The listing builds one solid part. Answer for the finished solid, in the listing's coordinates (mm). A direction names the side the tool comes from. Coordinates: 2 decimals unless noted, no trailing zeros. Loops run counter-clockwise (first coordinate to the right, second up) from the corner with the lowest first, then second, coordinate; pieces in that order, holes last. Notation, with made-up numbers: M 64.5,-28 L 68.5,-28 A10 ccw 68.5,-22 Z; hole C -14.5,54.5 d1. An arc over 180 degrees is marked long. Answer as CSV lines item,"result". Start each with the question number.
```python
from build123d import *

# Parameters (mm, degrees)
SKETCH2_R               = 20
BOSS_EXTRUDE1_DEPTH     = 20
SKETCH3_R               = 63.245553203
SKETCH3_R_2             = 55
CUT_EXTRUDE1_DEPTH      = 101
CUT_EXTRUDE1_DEPTH_BACK = 10


with BuildPart() as part:
    # Sketch1 → Revolve1 (revolve)
    with BuildSketch(Plane(origin=(0, 0, 0), x_dir=(1, 0, 0), z_dir=(0, 1, 0))):
        Polygon((70, -780), (70, -730), (60, -730), (60, -40), (0, -40), (0, -60), (45, -60), (45, -700), (25, -700), (25, -780), align=None)
    revolve(axis=Axis((0, 0, 0), (0, 0, 1)))

    # Sketch2 → Boss-Extrude1 (add, symmetric)
    with BuildSketch(Plane(origin=(0, 0, 0), x_dir=(1, 0, 0), z_dir=(0, 1, 0))):
        with BuildLine():
            Line((60, -40), (60, 0))
            ThreePointArc((60, 0), (0, 60), (-60, 0))
            Line((-60, 0), (-60, -40))
            Line((-60, -40), (60, -40))
        make_face()
        Circle(SKETCH2_R, mode=Mode.SUBTRACT)
    extrude(amount=BOSS_EXTRUDE1_DEPTH, both=True)

    # Sketch3 → Cut-Extrude1 (cut, two sides)
    with BuildSketch(Plane(origin=(0, 0, 40), x_dir=(-1, 0, 0), z_dir=(0, 0, -1))) as cut_extrude1_sk:
        Circle(SKETCH3_R)
        Circle(SKETCH3_R_2, mode=Mode.SUBTRACT)
    extrude(amount=CUT_EXTRUDE1_DEPTH, mode=Mode.SUBTRACT)
    extrude(cut_extrude1_sk.sketch, amount=-CUT_EXTRUDE1_DEPTH_BACK, mode=Mode.SUBTRACT)


solid = part.part
```
Item 1: For faces 4 (the face through (-1, 20, -22)), 5 (the face through (-59.94, 2.64, 385.24)), 6 (the face through (-1, -33, 40)), 7 (the face through (19, -19, 700)), determine the directions among +Z, -Z, +X, -X, +Y, -Y from which every point of the face is accessible in a straight line to the end or side of a thin tool.
Item 2: Section D-D on z = 138 is taken. Determine the outline of the cut face in (x, y).
Item 3: Section B-B on z = 0 is taken. Determine the outline of the cut face in (x, y), then the cut area to 3 significant figures.
Item 4: Consider line 1 (X direction, y = -1.5, z = 0); line 2 (Z direction, x = 16, y = -38); line 3 (Y direction, x = 0, z = 479). Determine where each line is inside the solid, lowest interval first.
Item 5: Each of these flat-tipped pins is pushed along its axis until it touches: P1, Ø12, axis at y = -36.5, z = 515.5, coming from the +X side; P2, Ø8, axis at x = -18.5, z = 228.5, coming from the +Y side; P3, Ø1.5, axis at y = -50.5, z = 662, coming from the -X side. Where does it stop, or does it pass through?
Item 6: Section A-A on x = 0 is taken. Determine the outline of the cut face in (y, z), then the cut area to 3 significant figures.
Item 7: Section C-C on y = 0 is taken. Determine the outline of the cut face in (x, z).
Item 8: For a pull along X with two mould halves and no side action, classify faces 1 (the face through (-55.55, -42.594, 754.65)), 2 (the face through (20.765, -39.923, 384.48)), 3 (the face through (-26, -49, 50)) as pulls with the +X half, pulls with the -X half, needs draft (parallel to the pull), parting line crosses it, or undercut.
Results are:
1,face 4,"-Z, +X, -X, +Y"
1,face 5,"-Z"
1,face 6,"-Z, +X, -X, -Y"
1,face 7,"none"
2,outline,"C 0,0 d120; hole C 0,0 d90"
3,outline,"M -51.23,-20 L -20,-20 L -20,20 L -51.23,20 A55 ccw Z; M 20,-20 L 51.23,-20 A55 ccw 51.23,20 L 20,20 Z"
3,area,"2,700 mm²"
4,line 1,"-54.98 to -20, 20 to 54.98"
4,line 2,"40 to 60, 700 to 780"
4,line 3,"-60 to -45, 45 to 60"
5,P1,"x = 51.67"
5,P2,"y = 58.22"
5,P3,"x = -33.54"
6,outline,"M -70,730 L -60,730 L -60,50 L -55,50 L -55,40 L -20,40 L -20,20 L 20,20 L 20,40 L 55,40 L 55,50 L 60,50 L 60,730 L 70,730 L 70,780 L 25,780 L 25,700 L 45,700 L 45,60 L -45,60 L -45,700 L -25,700 L -25,780 L -70,780 Z; M -20,-60 L 20,-60 L 20,-20 L -20,-20 Z"
6,area,"30,500 mm²"
7,outline,"M -70,730 L -60,730 L -60,50 L -55,50 L -55,-23.98 A60 ccw 55,-23.98 L 55,50 L 60,50 L 60,730 L 70,730 L 70,780 L 25,780 L 25,700 L 45,700 L 45,60 L -45,60 L -45,700 L -25,700 L -25,780 L -70,780 Z; hole C 0,0 d40"
8,face 1,"parting line crosses it"
8,face 2,"undercut"
8,face 3,"needs draft"
